Autodesk Inventor part; units mm, degrees
ref_plane "YZ Plane" through (0, 0, 0) normal (1, 0, 0) x (0, 1, 0)
ref_plane "XZ Plane" through (0, 0, 0) normal (0, 1, 0) x (-1, 0, 0)
ref_plane "XY Plane" through (0, 0, 0) normal (0, 0, 1) x (1, 0, 0)
sketch "Sketch1" plane through (0, 0, 0) normal (0, 1, 0) x (-1, 0, 0)
  circle A0 centre (0, 0) radius 4.6
  circle A1 centre (0, 0) radius 5.5
  line L0 (0, 5.5) -> (7.5, 5.5)
  line L1 (7.5, 5.5) -> (7.5, -5.5)
  line L2 (7.5, -5.5) -> (0, -5.5)
  line L3 (0, -5.5) -> (0, 5.5)
  line L4 (7.5, 5.5) -> (2.5, 5.5)
  line L5 (2.5, 5.5) -> (2.5, 8.5)
  line L6 (2.5, 8.5) -> (7.5, 8.5)
  line L7 (7.5, 8.5) -> (7.5, 5.5)
  line L8 (7.5, -5.5) -> (2.5, -5.5)
  line L9 (2.5, -5.5) -> (2.5, -8.5)
  line L10 (2.5, -8.5) -> (7.5, -8.5)
  line L11 (7.5, -8.5) -> (7.5, -5.5)
  circle A2 centre (0, 0) radius 7.5
  point P0 (2.5, -5.5)
  point P1 (2.5, 7.0711)
  point P2 (2.5, -7.0711)
  dimension "d1" = 11
  dimension "d0" = 9.2
  dimension "d2" = 5
  dimension "d3" = 3
  dimension "d4" = 5
  dimension "d5" = 3
extrude "Extrusion1" add sketch "Sketch1" along normal blind 7 contours A0 L3 A1 | A0 L3 A1 | L0 A2 L2 A1 | A1 L2 L9 A2 L5 L0 | L5 A2 L0 | L2 A2 L9 | A2 L5 L6 L7 L0 | L0 L1 A2 | A2 L1 L2 | L2 L11 L10 L9 A2
fillet "Fillet1" radius 3.175 2 edges at (-2.5, 3.5, -7.0711) (-2.5, 3.5, 7.0711)
sketch "Sketch2" plane through (-7.5, 0, -8.5) normal (-1, 0, 0) x (0, 0, 1)
  line L0 (0, 7) -> (17, 7)
  line L1 (0, 7) -> (3.5, 7)
  line L2 (3.5, 7) -> (13.5, 7)
  line L3 (3.5, 7) -> (3.5, 3.5)
  line L4 (0, 0) -> (17, 0)
  line L5 (13.5, 7) -> (13.5, 3.5)
  circle A0 centre (3.5, 3.5) radius 1
  circle A1 centre (13.5, 3.5) radius 1
  point P0 (8.5, 0)
  dimension "d9" = 3.5
  dimension "d10" = 10
  dimension "d11" = 3.5
  dimension "d12" = 3.5
  dimension "d13" = 2
  dimension "d14" = 2
extrude "Extrusion2" cut sketch "Sketch2" against normal blind 7
properties part number "screw_support"
The listing builds one solid part. Answer for the finished solid, in the listing's coordinates (mm). A direction names the side the tool comes from. Coordinates: 2 decimals unless noted, no trailing zeros. Order: outer loops, then holes, each group sorted by start corner. A loop starts at its lowest first (then second) coordinate and runs counter-clockwise, first axis right, second up.
Q1. Consider line 1 (Y direction, x = -2.75, z = -5); line 2 (Z direction, x = -3.5, y = 3.5); line 3 (X direction, y = 5, z = 2.5). Determine where each line is inside the solid, lowest interval first.
Q2. A cutting plane is placed at C-C, the plane x = 2.5. Write down the section's boundary in (y, z), and give its area (3 significant figures).
Q3. A cutting plane is placed at A-A, the plane z = 0. Write down the section's boundary in (x, y), and give its area (3 significant figures).
Q4. For a pull along Z with two mould halves and no side action, classify faces 1 (the face through (-4.049, 3.8, 5.954)), 2 (the face through (-5, 0, 0)), 3 (the face through (-1.438, 3.451, 7.756)) as pulls with the +Z half, pulls with the -Z half, needs draft (parallel to the pull), parting line crosses it, or undercut.
Q5. Which of the six approach directions +Z, -Z, +X, -X, +Y, -Y give full straight-line access (tool end or side, diameter ignored) to faces 4 (the face through (-4, 3.5, -6)), 5 (the face through (-5, 3, 8.5))?
Q6. A cutting plane is placed at B-B, the plane y = 6. Write down the section's boundary in (x, z) (3 decimals).
Q7. Given P1, Ø1.8, axis at y = 3.5, z = 5, coming from the +X side; P2, Ø1, axis at x = 3, y = 6, coming from the -Z side; P3, Ø1.6, axis at y = 3.5, z = -5, coming from the +X side, each flat-ended and moving along its own axis, determine where each tip first touches the part or whether it passes through.
Q8. A cutting plane is placed at D-D, the plane x = -5.75. Write down the section's boundary in (y, z), and give its area (3 significant figures).
Answers follow:
1. line 1: y = 0 to 2.5, 4.5 to 7
1. line 2: z = -8.5 to -6, -4 to -2.98, 2.98 to 4, 6 to 8.5
1. line 3: x = -7.5 to -3.86, 3.86 to 7.07
2. outline: (0, -7.07) - (7, -7.07) - (7, -3.86) - (0, -3.86) - close; (0, 3.86) - (7, 3.86) - (7, 7.07) - (0, 7.07) - close
2. area: 44.9 mm2
3. outline: (-7.5, 0) - (-4.6, 0) - (-4.6, 7) - (-7.5, 7) - close; (4.6, 0) - (7.5, 0) - (7.5, 7) - (4.6, 7) - close
3. area: 40.6 mm2
4. face 1: undercut
4. face 2: needs draft
4. face 3: pulls with the +Z half
5. face 4: -X
5. face 5: +Z, +X, -X, +Y, -Y
6. outline: (-7.5, -8.5) - (-2.5, -8.5) arc R3.175 cw to (-0.13, -7.499) arc R7.5 ccw (long way) to (-0.13, 7.499) arc R3.175 cw to (-2.5, 8.5) - (-7.5, 8.5) - close; hole circle Ø9.2 at (0, 0)
7. P1: stops at x = 6.28
7. P2: stops at z = -7.07
7. P3: stops at x = 6.21
8. outline: (0, -8.5) - (7, -8.5) - (7, 8.5) - (0, 8.5) - close; hole circle Ø2 at (3.5, -5); hole circle Ø2 at (3.5, 5)
8. area: 113 mm2
